Geometry: see drawing. Coordinates: mm, zero at the bounding-box minimum. A direction names the side the tool comes from. Coordinates: 2 decimals unless noted, no trailing zeros. Loops run counter-clockwise (first coordinate to the right, second up) from the corner with the lowest first, then second, coordinate; pieces in that order, holes last.
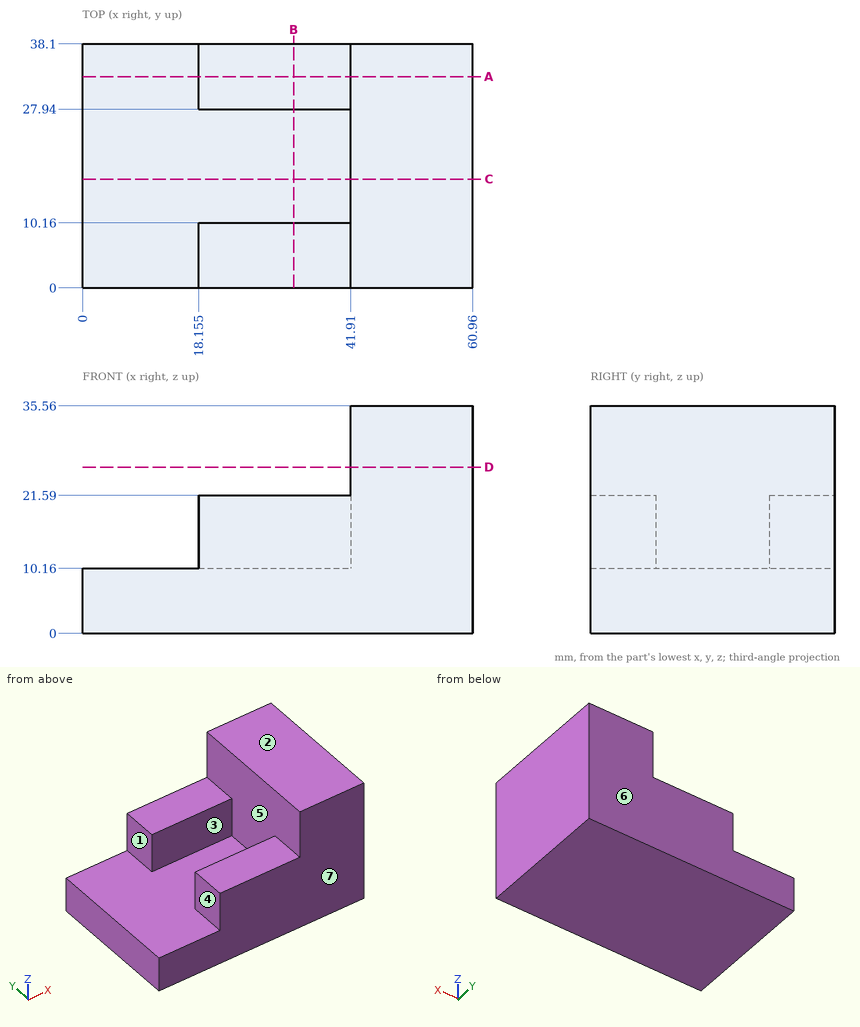
Item 1: Line query: L1, parallel to X at y = 11, z = 25.5; L2, parallel to Z at x = 16, y = 6; L3, parallel to X at y = 2, z = 17 (3 decimals). Output: solid intervals per line, ascending.
Result:
L1: x = 41.91 to 60.96
L2: z = 0 to 10.16
L3: x = 18.155 to 60.96
Item 2: Contact query for flat-ended pins moving along their axis: P1, Ø11, axis at x = 31.5, y = 4, coming from the +Z side; P2, Ø20.5, axis at y = 27.5, z = 29, coming from the -X side (3 decimals); P3, Ø8, axis at y = 19.5, z = 23, coming from the -X side; P4, Ø4, axis at x = 7.5, y = 13.5, coming from the -Z side. Output: stop coordinate, or through.
Result:
P1: stops at z = 21.59
P2: stops at x = 18.155
P3: stops at x = 41.91
P4: stops at z = 0
Item 3: Reachability of the marked faces 1, 2 and 3 from +Z, -Z, +X, -X, +Y, -Y: full face, straight path, thin tool, end or side. Return the list, or none.
Result:
face 1: +Z, -X, +Y, -Y
face 2: +Z, +X, -X, +Y, -Y
face 3: +Z, -X
Item 4: Section query B-B (x = 33). Output: boundary loops of the cut face in (y, z).
Result:
outline: (0, 0) - (38.1, 0) - (38.1, 21.59) - (27.94, 21.59) - (27.94, 10.16) - (10.16, 10.16) - (10.16, 21.59) - (0, 21.59) - close
Item 5: Section query D-D (z = 26). Output: boundary loops of the cut face in (x, y).
Result:
outline: (41.91, 0) - (60.96, 0) - (60.96, 38.1) - (41.91, 38.1) - close
Item 6: Mould query, pull axis Y, two halves, no side actions, for the marked faces 4, 5, 6 and 7. Classes: +Y half, -Y half, draft (parallel to the pull), parting line (faces both ways), or undercut.
Result:
face 4: draft
face 5: undercut
face 6: +Y half
face 7: -Y half
Item 7: Section query A-A (y = 33). Output: boundary loops of the cut face in (x, z) (3 decimals), then the cut area to 3 significant figures.
Result:
outline: (0, 0) - (60.96, 0) - (60.96, 35.56) - (41.91, 35.56) - (41.91, 21.59) - (18.155, 21.59) - (18.155, 10.16) - (0, 10.16) - close
area: 1,370 mm2
Item 8: Section query C-C (y = 17). Output: boundary loops of the cut face in (x, z), then the cut area to 3 significant figures.
Result:
outline: (0, 0) - (60.96, 0) - (60.96, 35.56) - (41.91, 35.56) - (41.91, 10.16) - (0, 10.16) - close
area: 1,100 mm2
